Source: three-view drawing plus pictorial views. Frame: mm from the lowest corner of the part. Coordinates: 2 decimals unless noted, no trailing zeros. Order: outer loops, then holes, each group sorted by start corner. A loop starts at its lowest first (then second) coordinate and runs counter-clockwise, first axis right, second up. Notation, with made-up numbers: (26, -31) - (65, -31) arc R15 ccw to (65, -10) - close; hole circle Ø10 at (86, -21). An arc over 180 degrees is marked (long way). Use a Markdown table: item, result. Add a question column.
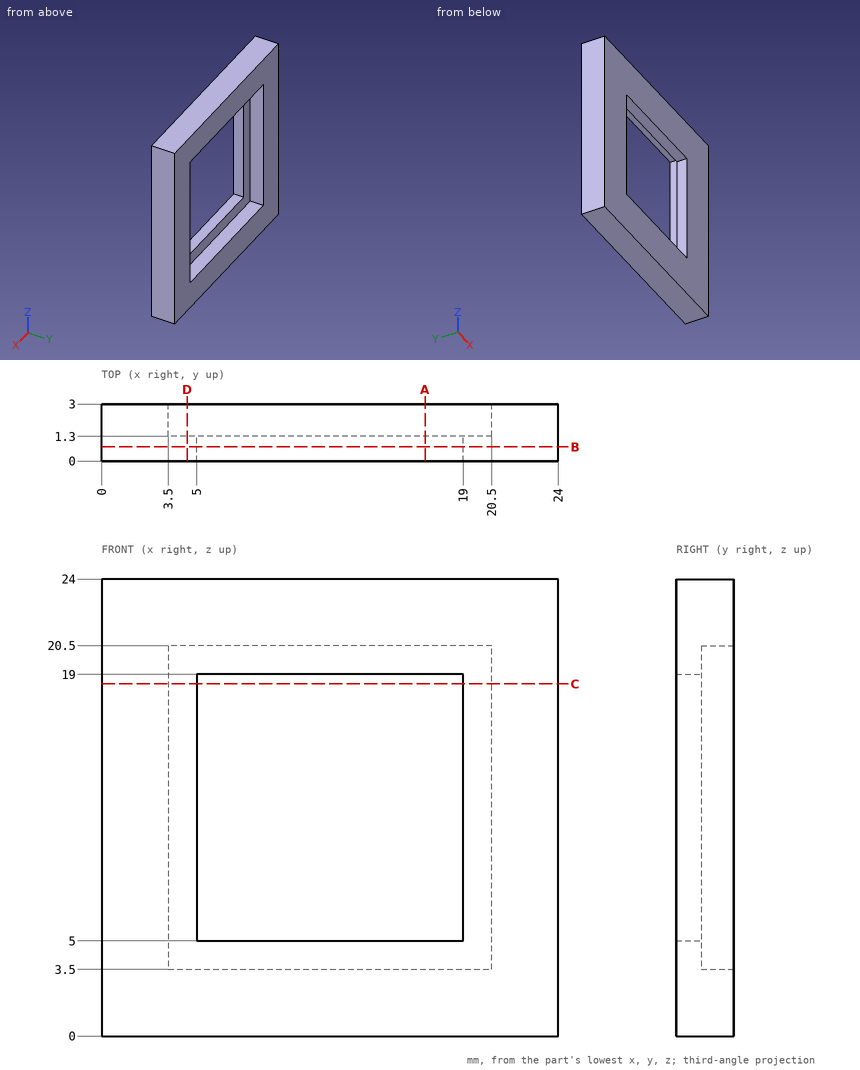
1) Section D-D (x = 4.5). Return loops of the section in (y, z).
2) Ray query, line 1 along X through (y, z) = (1.4, 11); line 2 along Z through (x, y) = (18.75, 0.9). Return the intervals inside material, ascending.
3) Pin query (flat end, axial travel): pin 1 (13.5 mm diameter, centred on x = 11, z = 11.5, fed in from +Y). Return the tip coordinate at first contact, or that it passes through.
4) Section C-C (z = 18.5). Return loops of the section in (x, y).
5) Section A-A (x = 17). Return loops of the section in (y, z), then the cut area to 3 significant figures.
6) Section B-B (y = 0.75). Return loops of the section in (x, z), then the cut area to 3 significant figures.
Values follow:
| question | item | result |
|---|---|---|
| 1 | outline | (0, 0) - (3, 0) - (3, 3.5) - (1.3, 3.5) - (1.3, 20.5) - (3, 20.5) - (3, 24) - (0, 24) - close |
| 2 | line 1 | x = 0 to 3.5, 20.5 to 24 |
| 2 | line 2 | z = 0 to 5, 19 to 24 |
| 3 | pin 1 | stops at y = 1.3 |
| 4 | outline | (0, 0) - (5, 0) - (5, 1.3) - (3.5, 1.3) - (3.5, 3) - (0, 3) - close; (19, 0) - (24, 0) - (24, 3) - (20.5, 3) - (20.5, 1.3) - (19, 1.3) - close |
| 5 | outline | (0, 0) - (3, 0) - (3, 3.5) - (1.3, 3.5) - (1.3, 5) - (0, 5) - close; (0, 19) - (1.3, 19) - (1.3, 20.5) - (3, 20.5) - (3, 24) - (0, 24) - close |
| 5 | area | 24.9 mm² |
| 6 | outline | (0, 0) - (24, 0) - (24, 24) - (0, 24) - close; hole (5, 5) - (19, 5) - (19, 19) - (5, 19) - close |
| 6 | area | 380 mm² |
